Read the model definition and answer for the solid it produces. Units are mm, in the model's axes. A direction names the side the tool comes from. Give positions to 0.01 mm unless a question says otherwise; leave off trailing zeros. Loops run counter-clockwise (first coordinate to the right, second up) from the corner with the lowest first, then second, coordinate; pieces in that order, holes last. Notation, with made-up numbers: (17.25, 10.25) - (35.25, 10.25) arc R12 cw to (35.25, 29.25) - close; hole circle Ø1 at (13, -17.75). An arc over 180 degrees is marked (long way). Put each result on its own line as item: value. Start each with the question number.
1. Given pin 1 Ø2 at (x, z) = (24, 2.5) entering from -Y; pin 2 Ø2 at (y, z) = (-32.5, 3.5) entering from -X; pin 3 Ø1 at (x, z) = (25.5, 1.5) entering from -Y, each flat-ended and moving along its own axis, determine where each tip first touches the part or whether it passes through.
2. A cutting plane is placed at B-B, the plane z = 2.5. Determine the outline of the cut face in (x, y), plus the area to 3 significant figures.
3. A cutting plane is placed at A-A, the plane x = 16. Determine the outline of the cut face in (y, z), plus the area to 3 significant figures.
4. A cutting plane is placed at D-D, the plane x = 36.5. Determine the outline of the cut face in (y, z).
5. For faces 5 (the cylindrical face through (21.91, -20.6, 3.22)), 6 (the flat face through (31.51, -40.52, 3.13)), determine the directions among +Z, -Z, +X, -X, +Y, -Y from which every point of the face is accessible in a straight line to the end or side of a thin tool.
6. A cutting plane is placed at C-C, the plane y = -37. Determine the outline of the cut face in (x, z), plus the area to 3 significant figures.
7. For a pull along X with two mould halves and no side action, classify faces 1 (the flat face through (0, -19.05, 3)), 2 (the cylindrical face through (51.311, -7.397, 3.131)), 3 (the flat face through (-31.339, -40.706, 3.131)), 4 (the flat face through (-1, 0, 3)) as released by +X, released by -X, zero draft, split by the parting line, or undercut.
8. Consider L1, parallel to X at y = -39, z = 1.25; L2, parallel to X at y = -41, z = 2.5; L3, parallel to Y at x = -0.5, z = 5. Determine where each line is inside the solid, lowest interval first. Write a range as from..to.
```python
from build123d import *

# Parameters (mm, degrees)
BOSS_EXTRUDE2_DEPTH = 6.35
CHAMFER1_SIZE       = 17.62
CHAMFER1_SIZE2      = 16.260294621
FILLET1_R           = 2.54
FILLET2_R           = 7.62


with BuildPart() as part:
    # Sketch1 → Boss-Extrude2 (new body)
    with BuildSketch(Plane.XY):
        with BuildLine():
            Line((0, -74.917600754), (-49.136391394, -21.278600827))
            ThreePointArc((-49.136391394, -21.278600827), (-51.395766113, -7.584251301), (-39.7716913, 0))
            Line((-39.7716913, 0), (0, 0))
            Line((0, 0), (39.7716913, 0))
            ThreePointArc((39.7716913, 0), (51.395766113, -7.584251301), (49.136391394, -21.278600827))
            Line((49.136391394, -21.278600827), (0, -74.917600754))
        make_face()
        Polygon((0, -46.715449274), (25.343133643, -19.05), (0, -19.05), (-25.343133643, -19.05), align=None, mode=Mode.SUBTRACT)
    extrude(amount=BOSS_EXTRUDE2_DEPTH)

    # Chamfer1
    chamfer1_edges = [part.edges().sort_by_distance(p)[0] for p in [
        (0, -74.917600754, 3.175),
    ]]
    chamfer1_side = [part.faces().sort_by_distance(p)[0] for p in [
        (-24.568195697, -48.098100791, 3.175),
    ]]
    chamfer(chamfer1_edges, length=CHAMFER1_SIZE, length2=CHAMFER1_SIZE2, reference=chamfer1_side[0])

    # Fillet1
    fillet1_edges = [part.edges().sort_by_distance(p)[0] for p in [
        (-25.343133643, -19.05, 3.175),
        (0, -46.715449274, 3.175),
        (25.343133643, -19.05, 3.175),
    ]]
    fillet(fillet1_edges, radius=FILLET1_R)

    # Fillet2
    fillet2_edges = [part.edges().sort_by_distance(p)[0] for p in [
        (10.98350999, -62.927617875, 3.175),
        (-11.901964297, -61.925001096, 3.175),
    ]]
    fillet(fillet2_edges, radius=FILLET2_R)


solid = part.part
```
Return value:
1. pin 1: stops at y = -49.81
1. pin 2: stops at x = -39.77
1. pin 3: stops at y = -47.63
2. outline: (-49.14, -21.28) - (-14.03, -59.6) arc R7.62 ccw to (-8.75, -62.06) - (7.43, -62.77) arc R7.62 ccw to (13.38, -60.31) - (49.14, -21.28) arc R12.7 ccw to (39.77, 0) - (-39.77, 0) arc R12.7 ccw to start; hole (-21.44, -23.31) - (-1.87, -44.67) arc R2.54 ccw to (1.87, -44.67) - (21.44, -23.31) arc R2.54 ccw to (19.57, -19.05) - (-19.57, -19.05) arc R2.54 ccw to start
2. area: 3,950 mm2
3. outline: (-57.45, 0) - (-29.25, 0) - (-29.25, 6.35) - (-57.45, 6.35) - close; (-19.05, 0) - (0, 0) - (0, 6.35) - (-19.05, 6.35) - close
3. area: 300 mm2
4. outline: (-35.07, 0) - (0, 0) - (0, 6.35) - (-35.07, 6.35) - close
5. face 5: +Z, -Z
5. face 6: +Z, -Z, +X, -Y
6. outline: (-34.73, 0) - (-8.9, 0) - (-8.9, 6.35) - (-34.73, 6.35) - close; (8.9, 0) - (34.73, 0) - (34.73, 6.35) - (8.9, 6.35) - close
6. area: 328 mm2
7. face 1: undercut
7. face 2: released by +X
7. face 3: released by -X
7. face 4: zero draft
8. L1: x = -32.9..-7.07, 7.07..32.9
8. L2: x = -31.07..-5.24, 5.24..31.07
8. L3: y = -62.42..-45.45, -19.05..0
